from build123d import *

# Parameters (mm, degrees)
BOSS_EXTRUDE1_DEPTH = 25
SKETCH3_R           = 4
CUT_EXTRUDE1_DEPTH  = 15
SKETCH4_R           = 15
BOSS_EXTRUDE2_DEPTH = 3
SKETCH5_R           = 7.5
BOSS_EXTRUDE3_DEPTH = 213


with BuildPart() as part:
    # Sketch1 → Boss-Extrude1 (new body)
    with BuildSketch(Plane(origin=(0, 0, 0), x_dir=(1, 0, 0), z_dir=(0, 1, 0))):
        with BuildLine():
            Line((-25, 55.5), (-88.782047704, 20.180509757))
            ThreePointArc((-88.782047704, 20.180509757), (-92.710355788, 17.967308971), (-96.105195929, 15))
            Line((-96.105195929, 15), (-109.105195929, 15))
            Line((-109.105195929, 15), (-109.105195929, 1))
            Line((-109.105195929, 1), (-95.968719423, 1))
            ThreePointArc((-95.968719423, 1), (-64, 0), (-95.968719423, -1))
            Line((-95.968719423, -1), (-109.105195929, -1))
            Line((-109.105195929, -1), (-109.105195929, -15))
            Line((-109.105195929, -15), (-96.105195929, -15))
            ThreePointArc((-96.105195929, -15), (-86.625068957, -20.987753506), (-75.425325161, -21.527881597))
            Line((-75.425325161, -21.527881597), (0, -5.5))
            Line((0, -5.5), (75.425325161, -21.527881597))
            ThreePointArc((75.425325161, -21.527881597), (86.625068957, -20.987753506), (96.105195929, -15))
            Line((96.105195929, -15), (109.105195929, -15))
            Line((109.105195929, -15), (109.105195929, -1))
            Line((109.105195929, -1), (95.968719423, -1))
            ThreePointArc((95.968719423, -1), (64, 0), (95.968719423, 1))
            Line((95.968719423, 1), (109.105195929, 1))
            Line((109.105195929, 1), (109.105195929, 15))
            Line((109.105195929, 15), (96.105195929, 15))
            ThreePointArc((96.105195929, 15), (92.710355788, 17.967308971), (88.782047704, 20.180509757))
            Line((88.782047704, 20.180509757), (25, 55.5))
            Line((25, 55.5), (1, 55.5))
            Line((1, 55.5), (-1, 55.5))
            Line((-1, 55.5), (-25, 55.5))
        make_face()
    extrude(amount=BOSS_EXTRUDE1_DEPTH)

    # Sketch3 → Cut-Extrude1 (cut, symmetric)
    with BuildSketch(Plane.XY):
        with Locations((-102.605195929, 12.5)):
            Circle(SKETCH3_R)
        with Locations(Location((102.605195929, 12.5, 0), (0, 0, 180))):
            Circle(SKETCH3_R)
    extrude(amount=CUT_EXTRUDE1_DEPTH, both=True, mode=Mode.SUBTRACT)

    # Sketch4 → Boss-Extrude2 (add)
    with BuildSketch(Plane(origin=(0, 25, 0), x_dir=(1, 0, 0), z_dir=(0, 1, 0))):
        with Locations(Location((0, 26, 0), (0, 0, 270))):
            Circle(SKETCH4_R)
    extrude(amount=BOSS_EXTRUDE2_DEPTH)

    # Sketch5 → Boss-Extrude3 (add)
    with BuildSketch(Plane(origin=(0, 28, 0), x_dir=(1, 0, 0), z_dir=(0, 1, 0))):
        with Locations(Location((0, 26, 0), (0, 0, 270))):
            Circle(SKETCH5_R)
    extrude(amount=BOSS_EXTRUDE3_DEPTH)


solid = part.part
Read the model definition and answer for the solid it produces. Units are mm, in the model's axes. A direction names the side the tool comes from. Coordinates: 2 decimals unless noted, no trailing zeros. Order: outer loops, then holes, each group sorted by start corner. A loop starts at its lowest first (then second) coordinate and runs counter-clockwise, first axis right, second up. Notation, with made-up numbers: M -22.5,-1.75 L 5.5,-1.75 A15 cw 5.5,22.25 Z; hole C -29.75,-38.5 d5. An arc over 180 degrees is marked long. Put each result on its own line as item: value. Start each with the question number.
Item 1: For faces 5 (the face through (0.66, 26.479, -40.985)), 6 (the face through (-106, 10, 15)), 7 (the face through (37.18, 12.32, 13.4)), determine the directions among +Z, -Z, +X, -X, +Y, -Y from which every point of the face is accessible in a straight line to the end or side of a thin tool.
Item 2: Section D-D, the plane y = 12.5 is taken. Count the separate pieces of the cut face and the enclosed holes in it, plus the area to 3 significant figures.
Item 3: The mould has two halves that part along X. Classify faces 1 (the face through (92.76, 12.32, -17.93)), 2 (the face through (-105.553, 15.203, -7.902)), 3 (the face through (-56.44, 12.32, -38.09)), 4 (the face through (-99.5, 9.5, 1)): +X half, -X half, draft (parallel to the pull), parting line (faces both ways), or undercut.
Item 4: Consider probe 1 along Z at (x, y) = (80, 8.75); probe 2 along X at (y, z) = (12, 5); probe 3 along X at (y, z) = (224.5, -25.5). Determine where each line is inside the solid, lowest interval first. Write a range as [from, to].
Item 5: Section B-B, the plane x = -80 is taken. Determine the outline of the cut face in (y, z), plus the area to 3 significant figures.
Item 6: Given pin 1 Ø5 at (x, z) = (24, -8.5) entering from +Y; pin 2 Ø10.5 at (x, y) = (103, 8) entering from -Z; pin 3 Ø6 at (y, z) = (130.5, -15) entering from -X; pin 4 Ø10.5 at (x, y) = (-105, 15) entering from +Z, each flat-ended and moving along its own axis, determine where each tip first touches the part or whether it passes through.
Item 7: Section C-C, the plane z = -26 is taken. Determine the outline of the cut face in (x, y).
Item 8: Section A-A, the plane z = -4 is taken. Determine the outline of the cut face in (x, y), plus the area to 3 significant figures.
Computed:
1. face 5: +Y
1. face 6: +Z, -X, +Y, -Y
1. face 7: +Z, +Y, -Y
2. separate pieces: 5
2. enclosed holes: 0
2. area: 9,410 mm2
3. face 1: +X half
3. face 2: undercut
3. face 3: -X half
3. face 4: draft
4. probe 1: z = [-25.04, -16], [16, 22.01]
4. probe 2: x = [-109.11, -106.57], [-98.64, -95.2], [-64.8, 64.8], [95.2, 98.64], [106.57, 109.11]
4. probe 3: x = [-7.48, 7.48]
5. outline: M 0,-25.04 L 25,-25.04 L 25,-16 L 0,-16 Z; M 0,16 L 25,16 L 25,22.01 L 0,22.01 Z
5. area: 376 mm2
6. pin 1: stops at y = 25
6. pin 2: stops at z = -15
6. pin 3: passes through
6. pin 4: stops at z = 15
7. outline: M -78.27,0 L 78.27,0 L 78.27,25 L 15,25 L 15,28 L 7.5,28 L 7.5,241 L -7.5,241 L -7.5,28 L -15,28 L -15,25 L -78.27,25 Z
8. outline: M -109.11,0 L -95.49,0 L -95.49,25 L -109.11,25 Z; M -64.51,0 L 64.51,0 L 64.51,25 L -64.51,25 Z; M 95.49,0 L 109.11,0 L 109.11,25 L 95.49,25 Z; hole C -102.61,12.5 d8; hole C 102.61,12.5 d8
8. area: 3,810 mm2
